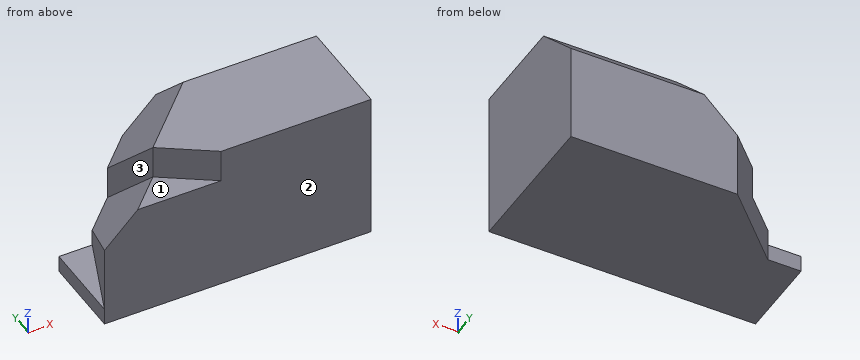
```python
from build123d import *

# Parameters (mm, degrees)
BOSS_EXTRUDE1_DEPTH = 9
CUT_EXTRUDE1_DEPTH  = 8
CUT_EXTRUDE2_DEPTH  = 8
CUT_EXTRUDE3_DEPTH  = 8
CUT_EXTRUDE4_DEPTH  = 8
CUT_EXTRUDE5_DEPTH  = 2


with BuildPart() as part:
    # Sketch1 → Boss-Extrude1 (new body)
    with BuildSketch(Plane.XY):
        Polygon((-6, 0.5), (-8, 0.5), (-8, -4.5), (8, -4.5), (8, 4.5), (-2, 4.5), align=None)
    extrude(amount=BOSS_EXTRUDE1_DEPTH)

    # Sketch2 → Cut-Extrude1 (cut)
    with BuildSketch(Plane.XY.offset(9)):
        Polygon((-8, 0.5), (-6, 0.5), (-8, -4.5), align=None)
    extrude(amount=-CUT_EXTRUDE1_DEPTH, mode=Mode.SUBTRACT)

    # 3DSketch1 → Cut-Extrude2 (cut, along a direction that is not the sketch's normal)
    with BuildSketch(Plane(origin=(-8, -4.5, 5), x_dir=(0.464990554975277, 0.8137334712067351, -0.3487429162314579), z_dir=(0.5773502691896258, -0.5773502691896257, -0.5773502691896258))):
        Polygon((0, 0), (6.044877215, -1.208080899), (8.602325267, 0), (2.78994333, 4.026936331), (0.232495277, 2.818855432), align=None)
    extrude(amount=-CUT_EXTRUDE2_DEPTH, dir=(0, 0, -1), mode=Mode.SUBTRACT)

    # 3DSketch2 → Cut-Extrude3 (cut, along a direction that is not the sketch's normal)
    with BuildSketch(Plane(origin=(-4, -2.5, 9), x_dir=(0.2264554068289193, 0.7925939239012171, -0.5661385170722979), z_dir=(0.5773502691896256, -0.5773502691896258, -0.5773502691896258))):
        Polygon((0, 0), (6.793662205, -1.961161351), (8.831760866, 0), (8.152394646, 2.745625892), (4.076197323, 3.922322703), align=None)
    extrude(amount=-CUT_EXTRUDE3_DEPTH, dir=(0, 0, -1), mode=Mode.SUBTRACT)

    # Sketch3 → Cut-Extrude4 (cut)
    with BuildSketch(Plane.ZY):
        Polygon((9, 1.5), (6, 4.5), (9, 4.5), align=None)
    extrude(amount=-CUT_EXTRUDE4_DEPTH, mode=Mode.SUBTRACT)

    # Sketch4 → Cut-Extrude5 (cut)
    with BuildSketch(Plane.XY.offset(9)):
        Polygon((-4, -2.5), (-1, -4.5), (-6, -4.5), align=None)
    extrude(amount=-CUT_EXTRUDE5_DEPTH, mode=Mode.SUBTRACT)


solid = part.part
```
CAD build for the part. Positions are in the model's coordinates, mm. Face numbers are marked on the shaded views. A direction names the side the tool comes from. Give positions to 0.01 mm unless a question says otherwise; leave off trailing zeros. Write each loop counter-clockwise with the first axis right and the second up, starting at its lowest first coordinate (ties: lowest second). Pieces come first, ordered by that corner, then holes. Notation, with made-up numbers: M 2,46 L 37,46 A15 cw 37,63 Z; hole C 10,-24.5 d6. An arc over 180 degrees is marked long. Return JSON: item names as keys, results as strings. Group by question number.
(1) Flat gauge pins, fed straight in: pin 1 Ø4 at (y, z) = (0.5, 7) entering from -X; pin 2 Ø2 at (x, y) = (-6.5, -1.5) entering from +Z; pin 3 Ø0.8 at (x, z) = (-6.5, 0.5) entering from +Y. Where does each tip first touch, or does it go through?
(2) Band-saw the part on C-C (x = -0.5). Give the cut face in (y, z).
(3) Drill centre lines: L1, parallel to X at y = 1.5, z = 4; L2, parallel to Z at x = -3, y = 2.5; L3, parallel to X at y = -2, z = 4.5. Where is each one in solid material? Low to high. Write a range as [from, to].
(4) Band-saw the part on A-A (y = 3). Give the cut face in (x, z), and give its area (3 significant figures).
(5) 3-axis set-ups, long thin cutter, end or side, ignore diameter. For the marked faces 1, 2 and 3: which of +Z, -Z, +X, -X, +Y, -Y reach the whole face in a straight line?
(6) Band-saw the part on D-D (y = -2.25). Give the cut face in (x, z).
(7) Band-saw the part on B-B (z = 8.25). Give the cut face in (x, y), and give its area (3 significant figures).
Entries:
{
 "1": {"pin 1": "stops at x = -4", "pin 2": "stops at z = 4.91", "pin 3": "stops at y = 0.5"},
 "2": {"outline": "M -4.5,0 L 4.5,0 L 4.5,5.5 L 1,9 L -4.5,9 Z"},
 "3": {"L1": "x = [-4, 8]", "L2": "z = [0, 5]", "L3": "x = [-6, 8]"},
 "4": {"outline": "M -3.5,0 L 8,0 L 8,7.5 L 0,7.5 L -3.5,4 Z", "area": "80.1 mm^2"},
 "5": {"face 1": "+Z, -X, -Y", "face 2": "+Z, -Z, +X, -X, -Y", "face 3": "+Z, -X, +Y"},
 "6": {"outline": "M -8,0 L 8,0 L 8,9 L -3.75,9 L -4,8.75 L -4,6.75 L -7.1,3.65 L -7.1,1 L -8,1 Z"},
 "7": {"outline": "M -4,-2.5 L -1,-4.5 L 8,-4.5 L 8,2.25 L 0,2.25 L -4,-1.75 Z", "area": "70.0 mm^2"}
}
